Could you check a few things on this model? Use its own coordinates, in mm. Face numbers are marked on the shaded views. A direction names the side the tool comes from. Round coordinates to 2 decimals unless told otherwise and drop trailing zeros. Loops run counter-clockwise (first coordinate to the right, second up) from the corner with the lowest first, then second, coordinate; pieces in that order, holes last. Notation, with made-up numbers: (85.25, 61.5) - (108.25, 61.5) arc R25 ccw to (108.25, 87.5) - close; hole circle Ø4 at (5.5, 64). An arc over 180 degrees is marked (long way). Answer as CSV lines item,"result". Start each with the question number.
1) Suppose I cut it at C-C, the plane x = 6. Write out the boundary of the cut face in (y, z), then the cut area to 3 significant figures.
2) Please list where these lines run through material, in increasing order: line 1 along X through (y, z) = (4.5, 8.5); line 2 along X through (y, z) = (31.95, 25); line 3 along Y through (x, z) = (20, 5).
3) Suppose I cut it at D-D, the plane z = 36.5. Write out the boundary of the cut face in (x, y).
4) We'd pull the mould along X, two halves only. Please class the marked faces 1, 2 and 3: pulls with the +X half, pulls with the -X half, needs draft (parallel to the pull), parting line crosses it, or undercut.
5) Which directions (+Z, -Z, +X, -X, +Y, -Y) give clear straight access to the entire face, cutting with the end or side of a thin tool? Please do the marked faces 4 and 5.
6) Suppose I cut it at B-B, the plane z = 25. Write out the boundary of the cut face in (x, y).
7) Suppose I cut it at A-A, the plane y = 15. Write out the boundary of the cut face in (x, z).
8) I'm going to push flat-ended pins straight in: pin 1 Ø3 at (x, z) = (9, 9) entering from +Y; pin 2 Ø6 at (x, z) = (-4.5, 30.5) entering from -Y. Where does each tip first touch, or does it pass through?
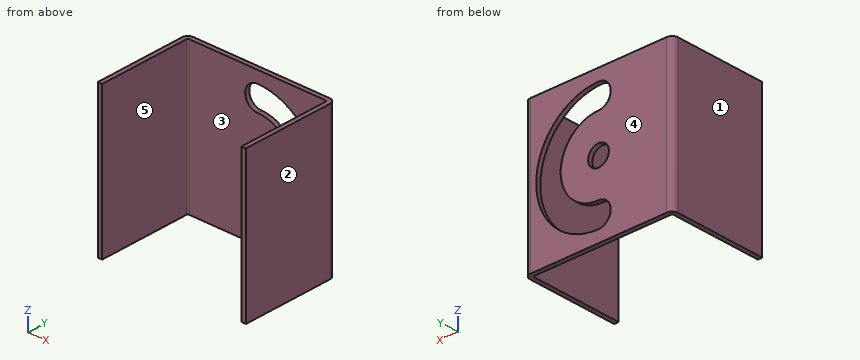
```python
from build123d import *

# Parameters (mm, degrees)
BASE_FLANGE1_DEPTH = 50
SKETCH2_R          = 3.5
CUT_EXTRUDE1_DEPTH = 10
CUT_EXTRUDE2_DEPTH = 3


# Sheet-metal steps are written as plain solids
with BuildPart() as part:
    # Sketch1 → Base-Flange1 (new body)
    with BuildSketch(Plane.XY):
        with BuildLine():
            Line((-25, 0), (-25, 30.930870366))
            ThreePointArc((-25, 30.930870366), (-24.414213562, 32.345083928), (-23, 32.930870366))
            Line((-23, 32.930870366), (23, 32.930870366))
            ThreePointArc((23, 32.930870366), (24.414213562, 32.345083928), (25, 30.930870366))
            Line((25, 30.930870366), (25, 0))
            Line((25, 0), (23.5, 0))
            Line((23.5, 0), (23.5, 30.930870366))
            ThreePointArc((23.5, 30.930870366), (23.353553391, 31.284423757), (23, 31.430870366))
            Line((23, 31.430870366), (-23, 31.430870366))
            ThreePointArc((-23, 31.430870366), (-23.353553391, 31.284423757), (-23.5, 30.930870366))
            Line((-23.5, 30.930870366), (-23.5, 0))
            Line((-23.5, 0), (-25, 0))
        make_face()
    extrude(amount=BASE_FLANGE1_DEPTH)

    # Sketch2 → Cut-Extrude1 (cut)
    with BuildSketch(Plane(origin=(0, 32.930870366, 0), x_dir=(1, 0, 0), z_dir=(0, 1, 0))):
        with Locations(Location((0, -25, 0), (0, 0, 270))):
            Circle(SKETCH2_R)
    extrude(amount=-CUT_EXTRUDE1_DEPTH, mode=Mode.SUBTRACT)

    # Sketch3 → Cut-Extrude2 (cut)
    with BuildSketch(Plane(origin=(0, 32.930870366, 0), x_dir=(1, 0, 0), z_dir=(0, 1, 0))):
        with BuildLine():
            ThreePointArc((0, -37.783779882), (12.783779882, -25), (0, -12.216220118))
            ThreePointArc((0, -12.216220118), (-4.117379141, -8.098840977), (0, -3.981461837))
            ThreePointArc((0, -3.981461837), (21.018538163, -25), (0, -46.018538163))
            ThreePointArc((0, -46.018538163), (-4.117379141, -41.901159023), (0, -37.783779882))
        make_face()
    extrude(amount=-CUT_EXTRUDE2_DEPTH, mode=Mode.SUBTRACT)


solid = part.part
```
Filled sheet:
1,outline,"(31.43, 0) - (32.93, 0) - (32.93, 4.86) - (31.43, 4.86) - close; (31.43, 13.71) - (32.93, 13.71) - (32.93, 36.29) - (31.43, 36.29) - close; (31.43, 45.14) - (32.93, 45.14) - (32.93, 50) - (31.43, 50) - close"
1,area,"48.4 mm²"
2,line 1,"-25 to -23.5, 23.5 to 25"
2,line 2,"-24.72 to -3.5, 3.5 to 12.78, 21.02 to 24.72"
2,line 3,"31.43 to 32.93"
3,outline,"(-25, 0) - (-23.5, 0) - (-23.5, 30.93) arc R0.5 cw to (-23, 31.43) - (5.58, 31.43) - (5.58, 32.93) - (-23, 32.93) arc R2 ccw to (-25, 30.93) - close; (17.59, 31.43) - (23, 31.43) arc R0.5 cw to (23.5, 30.93) - (23.5, 0) - (25, 0) - (25, 30.93) arc R2 ccw to (23, 32.93) - (17.59, 32.93) - close"
4,face 1,"pulls with the -X half"
4,face 2,"pulls with the +X half"
4,face 3,"undercut"
5,face 4,"+Z, -Z, +X, -X, +Y"
5,face 5,"+Z, -Z, -Y"
6,outline,"(-25, 0) - (-23.5, 0) - (-23.5, 30.93) arc R0.5 cw to (-23, 31.43) - (-3.5, 31.43) - (-3.5, 32.93) - (-23, 32.93) arc R2 ccw to (-25, 30.93) - close; (3.5, 31.43) - (12.78, 31.43) - (12.78, 32.93) - (3.5, 32.93) - close; (21.02, 31.43) - (23, 31.43) arc R0.5 cw to (23.5, 30.93) - (23.5, 0) - (25, 0) - (25, 30.93) arc R2 ccw to (23, 32.93) - (21.02, 32.93) - close"
7,outline,"(-25, 0) - (-23.5, 0) - (-23.5, 50) - (-25, 50) - close; (23.5, 0) - (25, 0) - (25, 50) - (23.5, 50) - close"
8,pin 1,"through"
8,pin 2,"y = 31.43"
